Autodesk Inventor part; units mm, degrees
ref_plane "YZ Plane" through (0, 0, 0) normal (1, 0, 0) x (0, 1, 0)
ref_plane "XZ Plane" through (0, 0, 0) normal (0, 1, 0) x (-1, 0, 0)
ref_plane "XY Plane" through (0, 0, 0) normal (0, 0, 1) x (1, 0, 0)
ref_plane "Arbeitsebene1" through (0, 0, 0) normal (0, 0, 1) x (1, 0, 0)
sketch "Skizze1" plane through (0, 0, 0) normal (0, 0, 1) x (1, 0, 0)
  line L0 (-29, -22.45) -> (-29, 20.1)
  line L1 (-29.2058, 20.9837) -> (-32.4027, 27.4738)
  line L2 (-17.2708, 40.1383) -> (-31.7557, 29.9959)
  line L3 (-16.1236, 40.5) -> (16.1236, 40.5)
  line L4 (33.1958, 28.9875) -> (17.2708, 40.1383)
  line L5 (34.0411, 27.1762) -> (28.1661, -40.5)
  line L6 (28.1661, -40.5) -> (-28.0975, -40.5)
  line L7 (-28.0975, -40.5) -> (-29, -22.45)
  line L8 (-30.9975, -22.5499) -> (-30.095, -40.5999)
  line L9 (-28.0975, -42.5) -> (28.1661, -42.5)
  line L10 (30.1586, -40.673) -> (36.2833, 29.879)
  line L11 (35.4379, 31.6903) -> (20.5166, 42.1383)
  line L12 (19.3694, 42.5) -> (-19.3694, 42.5)
  line L13 (-20.5166, 42.1383) -> (-34.9783, 32.0121)
  line L14 (-35.6253, 29.4901) -> (-31.2058, 20.5179)
  line L15 (-31, 19.6342) -> (-31, -22.45)
  line L16 (-32.5225, 28.8486) -> (-28.5, 20.6823)
  line L17 (-28.5, 20.6823) -> (-28.5, -22.4375)
  line L18 (-28.5, -22.4375) -> (-27.6219, -40)
  line L19 (-27.6219, -40) -> (27.7076, -40)
  line L20 (27.7076, -40) -> (33.6178, 28.0816)
  line L21 (33.6178, 28.0816) -> (16.5966, 40)
  line L22 (16.5966, 40) -> (-16.5966, 40)
  line L23 (-16.5966, 40) -> (-32.5225, 28.8486)
  arc A0 (-29, 20.1) -> (-29.2058, 20.9837) centre (-31, 20.1) ccw
  arc A1 (-31.7557, 29.9959) -> (-32.4027, 27.4738) centre (-30.6085, 28.3576) ccw
  arc A2 (-16.1236, 40.5) -> (-17.2708, 40.1383) centre (-16.1236, 38.5) ccw
  arc A3 (17.2708, 40.1383) -> (16.1236, 40.5) centre (16.1236, 38.5) ccw
  arc A4 (34.0411, 27.1762) -> (33.1958, 28.9875) centre (32.0486, 27.3492) ccw
  arc A5 (-31, -22.45) -> (-30.9975, -22.5499) centre (-29, -22.45) ccw
  arc A6 (-30.095, -40.5999) -> (-28.0975, -42.5) centre (-28.0975, -40.5) ccw
  arc A7 (28.1661, -42.5) -> (30.1586, -40.673) centre (28.1661, -40.5) ccw
  arc A8 (36.2833, 29.879) -> (35.4379, 31.6903) centre (34.2907, 30.052) ccw
  arc A9 (20.5166, 42.1383) -> (19.3694, 42.5) centre (19.3694, 40.5) ccw
  arc A10 (-19.3694, 42.5) -> (-20.5166, 42.1383) centre (-19.3694, 40.5) ccw
  arc A11 (-34.9783, 32.0121) -> (-35.6253, 29.4901) centre (-33.8311, 30.3738) ccw
  arc A12 (-31, 19.6342) -> (-31.2058, 20.5179) centre (-33, 19.6342) ccw
  point P0 (0, 0)
  dimension "d2" = 0.5
extrude "Extrusion1" add sketch "Skizze1" against normal blind 2 contours L23 L22 L21 L20 L19 L18 L17 L16
sketch "Skizze2" plane through (0, 0, 0) normal (0, 0, 1) x (-1, 0, 0)
  point P0 (0, 0)
sketch "Skizze3" plane through (0, 0, 0) normal (0, 0, 1) x (1, 0, 0)
  line L0 (-29, -22.45) -> (-29, 20.1)
  line L1 (-29.2058, 20.9837) -> (-32.4027, 27.4738)
  line L2 (-17.2708, 40.1383) -> (-31.7557, 29.9959)
  line L3 (-16.1236, 40.5) -> (16.1236, 40.5)
  line L4 (33.1958, 28.9875) -> (17.2708, 40.1383)
  line L5 (34.0411, 27.1762) -> (28.1661, -40.5)
  line L6 (28.1661, -40.5) -> (-28.0975, -40.5)
  line L7 (-28.0975, -40.5) -> (-29, -22.45)
  line L8 (-30.9975, -22.5499) -> (-30.095, -40.5999)
  line L9 (-28.0975, -42.5) -> (28.1661, -42.5)
  line L10 (30.1586, -40.673) -> (36.2833, 29.879)
  line L11 (35.4379, 31.6903) -> (20.5166, 42.1383)
  line L12 (19.3694, 42.5) -> (-19.3694, 42.5)
  line L13 (-20.5166, 42.1383) -> (-34.9783, 32.0121)
  line L14 (-35.6253, 29.4901) -> (-31.2058, 20.5179)
  line L15 (-31, 19.6342) -> (-31, -22.45)
  arc A0 (-29, 20.1) -> (-29.2058, 20.9837) centre (-31, 20.1) ccw
  arc A1 (-31.7557, 29.9959) -> (-32.4027, 27.4738) centre (-30.6085, 28.3576) ccw
  arc A2 (-16.1236, 40.5) -> (-17.2708, 40.1383) centre (-16.1236, 38.5) ccw
  arc A3 (17.2708, 40.1383) -> (16.1236, 40.5) centre (16.1236, 38.5) ccw
  arc A4 (34.0411, 27.1762) -> (33.1958, 28.9875) centre (32.0486, 27.3492) ccw
  arc A5 (-31, -22.45) -> (-30.9975, -22.5499) centre (-29, -22.45) ccw
  arc A6 (-30.095, -40.5999) -> (-28.0975, -42.5) centre (-28.0975, -40.5) ccw
  arc A7 (28.1661, -42.5) -> (30.1586, -40.673) centre (28.1661, -40.5) ccw
  arc A8 (36.2833, 29.879) -> (35.4379, 31.6903) centre (34.2907, 30.052) ccw
  arc A9 (20.5166, 42.1383) -> (19.3694, 42.5) centre (19.3694, 40.5) ccw
  arc A10 (-19.3694, 42.5) -> (-20.5166, 42.1383) centre (-19.3694, 40.5) ccw
  arc A11 (-34.9783, 32.0121) -> (-35.6253, 29.4901) centre (-33.8311, 30.3738) ccw
  arc A12 (-31, 19.6342) -> (-31.2058, 20.5179) centre (-33, 19.6342) ccw
  point P0 (0, 0)
extrude "Extrusion2" add sketch "Skizze3" along normal blind 2 contours L0 A0 L1 A1 L2 A2 L3 A3 L4 A4 L5 L6 L7 | A5 L15 A12 L14 A11 L13 A10 L12 A9 L11 A8 L10 A7 L9 A6 L8
sketch "Skizze4" plane through (0, 0, 2) normal (0, 0, 1) x (1, 0, 0)
  circle A0 centre (-25.2, -36.5) radius 1.5
  circle A1 centre (25.2, -36.5) radius 1.5
  circle A2 centre (0, 30.5) radius 1.5
  point P0 (0, 0)
hole "Bohrung1" at (0, 30.5, 2) at (25.2, -36.5, 2) at (-25.2, -36.5, 2) direction (0, 0, -1) diameter 4.2 end through all
fillet "Rundung1" radius 2 6 edges at (27.7076, -40, -1) (-27.6219, -40, -1) (33.6178, 28.0816, -1) (16.5966, 40, -1) (-32.5225, 28.8486, -1) (-16.5966, 40, -1)
properties part number "Deckel_oberteil"
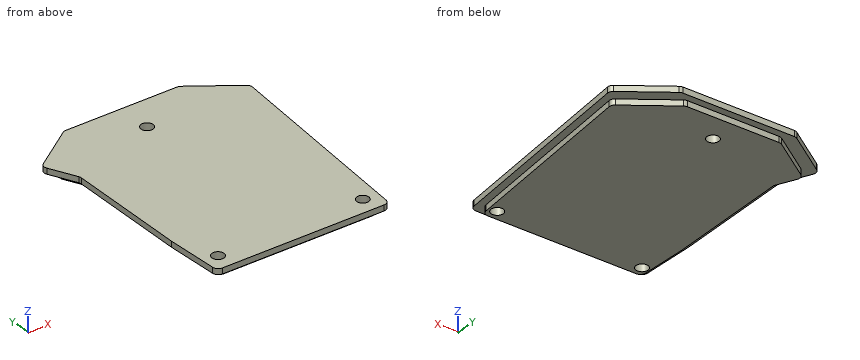
Here's how the part is built. I have some questions about the finished solid (model axes, mm). Coordinates: 2 decimals unless noted, no trailing zeros. Write each loop counter-clockwise with the first axis right and the second up, starting at its lowest first coordinate (ties: lowest second). Pieces come first, ordered by that corner, then holes.
Item 1: If I drill on line 1 (Y direction, x = 0, z = -0.85); line 2 (X direction, y = -36.5, z = -1.2); line 3 (X direction, y = -2, z = 0.35), over which ranges is the centre line in solid material (lowest first)?
Item 2: I want a section at B-B on z = 1.35. Count the separate pieces of the cut face and the enclosed holes in it, and give its area (3 significant figures).
Item 3: I want a section at D-D on y = -36.5. Write out the boundary of the cut face in (x, z).
Item 4: I want a section at C-C on x = -8. Write out the boundary of the cut face in (y, z).
Item 5: Will these pins go through, and if not, where does the flat tip stop? pin 1 (1.5 mm diameter, centred on y = -8.5, z = 1, fed in from -X); pin 2 (2 mm diameter, centred on y = -4, z = -1.5, fed in from -X); pin 3 (0.6 mm diameter, centred on x = -1, z = -1, fed in from +Y); pin 4 (3.5 mm diameter, centred on x = 25.2, y = -36.5, fed in from -Z).
Item 6: I want a section at A-A on x = 0. Write out the boundary of the cut face in (y, z).
Findings below:
1. line 1: y = -40 to 28.4, 32.6 to 40
1. line 2: x = -27.8 to -27.3, -23.1 to 23.1, 27.3 to 28.01
1. line 3: x = -31 to 33.52
2. separate pieces: 1
2. enclosed holes: 3
2. area: 5,340 mm2
3. outline: (-30.3, 0) - (-27.8, 0) - (-27.8, -2) - (-27.3, -2) - (-27.3, 2) - (-30.3, 2) - close; (-23.1, -2) - (23.1, -2) - (23.1, 2) - (-23.1, 2) - close; (27.3, -2) - (28.01, -2) - (28.01, 0) - (30.52, 0) - (30.52, 2) - (27.3, 2) - close
4. outline: (-42.5, 0) - (-40, 0) - (-40, -2) - (40, -2) - (40, 0) - (42.5, 0) - (42.5, 2) - (-42.5, 2) - close
5. pin 1: stops at x = -31
5. pin 2: stops at x = -28.5
5. pin 3: stops at y = 40
5. pin 4: passes through
6. outline: (-42.5, 0) - (-40, 0) - (-40, -2) - (28.4, -2) - (28.4, 2) - (-42.5, 2) - close; (32.6, -2) - (40, -2) - (40, 0) - (42.5, 0) - (42.5, 2) - (32.6, 2) - close
